```python
from build123d import *

# Parameters (mm, degrees)
DODANIE_WYCI_GNI_CIE1_DEPTH       = 2
WYCI_GNI_CIE_CIENKA_CIANKA1_DEPTH = 10
SZKIC3_R                          = 2.5
WYTNIJ_WYCI_GNI_CIE1_DEPTH        = 6


with BuildPart() as part:
    # Szkic1 → Dodanie-wyciągnięcie1 (new body)
    with BuildSketch(Plane(origin=(184.050171811, 0, -211.725502995), x_dir=(-0.75470958, 0, -0.656059029), z_dir=(0.656059029, 0, -0.75470958))):
        with BuildLine():
            Line((-818.756651821, -341.547090535), (-826.154339771, -317.666675693))
            Line((-826.154339771, -317.666675693), (-807.050007897, -311.748525334))
            Line((-807.050007897, -311.748525334), (-799.03222594, -337.630660478))
            add(Edge.make_bspline(
                [(-818.756651821, -341.547090535), (-812.651532186, -337.74352209), (-805.362739321, -336.365866813), (-799.03222594, -337.630660478)],
                knots=[0.197302397, 0.197302397, 0.197302397, 0.197302397, 0.33815529, 0.33815529, 0.33815529, 0.33815529], degree=3, weights=[0.522216299, 0.482629046, 0.495947227, 0.562170841]))
        make_face()
    extrude(amount=DODANIE_WYCI_GNI_CIE1_DEPTH)

    # Szkic2 → Wyciągnięcie-cienka ścianka1 (add)
    with BuildSketch(Plane(origin=(185.362289869, 0, -213.234922155), x_dir=(-0.75470958, 0, -0.656059029), z_dir=(0.656059029, 0, -0.75470958))):
        Polygon((-826.154339771, -317.666675693), (-807.050007897, -311.748525334), (-806.458192861, -313.658958521), (-825.562524735, -319.577108881), align=None)
    extrude(amount=WYCI_GNI_CIE_CIENKA_CIANKA1_DEPTH)

    # Szkic3 → Wytnij-wyciągnięcie1 (cut)
    with BuildSketch(Plane(origin=(-13.617240057, -58.24452258, -11.837286187), x_dir=(-0.974744215, 0.218850254, 0.044477883), z_dir=(-0.223324239, -0.955216594, -0.194132799))):
        with Locations((-839.308044037, -375.023490092)):
            Circle(SZKIC3_R)
    extrude(amount=-WYTNIJ_WYCI_GNI_CIE1_DEPTH, mode=Mode.SUBTRACT)


solid = part.part
```
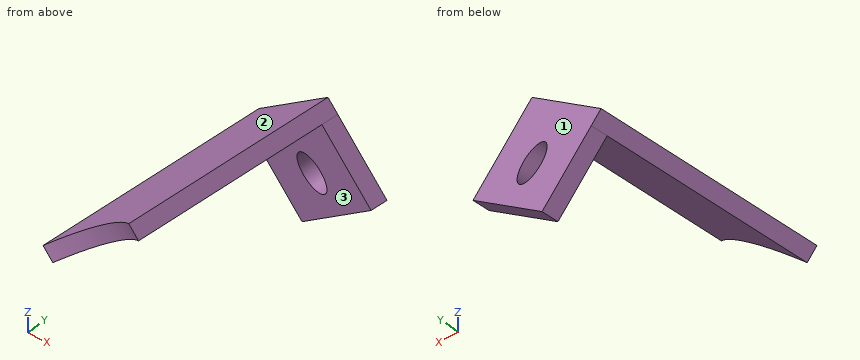
Here's how the part is built. I have some questions about the finished solid (model axes, mm). Face numbers are marked on the shaded views. Coordinates: 2 decimals unless noted, no trailing zeros. Loops run counter-clockwise (first coordinate to the right, second up) from the corner with the lowest first, then second, coordinate; pieces in that order, holes last. Notation, with made-up numbers: (63.5, 78.25) - (98.5, 78.25) arc R9 cw to (98.5, 87.25) - close; hole circle Ø5 at (-15.75, -10). An arc over 180 degrees is marked (long way). Return JSON: item names as keys, results as strings. Group by question number.
Item 1: We'd pull the mould along X, two halves only. Please class the marked faces 1, 2 and 3: +X half, -X half, draft (parallel to the pull), parting line (faces both ways), or undercut.
Item 2: I need wall thicknesses on line 1 (Z direction, x = 811.25, y = -318); line 2 (Z direction, x = 805.75, y = -328); line 3 (X direction, y = -323.75, z = 317). Which ranges of each line are inside material? Lowest first, please. Write a range as from..to.
Item 3: If we section it at B-B on z = 310.5: Write out the boundary of the cut face in (x, y), and give its area (3 significant figures).
Item 4: Will these pins go through, and if not, where does the flat tip stop? P1, Ø1.5, axis at x = 809.5, z = 319, coming from the +Y side; P2, Ø6, axis at y = -327, z = 320.5, coming from the -X side; P3, Ø3, axis at x = 803, z = 313, coming from the +Y side.
Item 5: If we section it at A-A on x = 811.75: Write out the boundary of the cut face in (y, z), and give its area (3 significant figures).
Calculated:
{
 "1": {"face 1": "+X half", "face 2": "-X half", "face 3": "undercut"},
 "2": {"line 1": "z = 317.59..325.87", "line 2": "z = 326.06..327.48", "line 3": "x = 792.28..795.33"},
 "3": {"outline": "(798.65, -313.66) - (803.09, -314.7) - (803.09, -312.6) - (799.44, -311.75) - close", "area": "8.47 mm^2"},
 "4": {"P1": "stops at y = -315.6", "P2": "stops at x = 792.85", "P3": "stops at y = -312.62"},
 "5": {"outline": "(-319.58, 324.55) - (-318.25, 318.03) - (-316.16, 318.03) - (-317.67, 325.46) - close", "area": "14.6 mm^2"}
}
